Geometry check sheet. Reference: the model listing, model coordinates, mm. A direction names the side the tool comes from. Round coordinates to 2 decimals unless told otherwise and drop trailing zeros. Write each loop counter-clockwise with the first axis right and the second up, starting at its lowest first coordinate (ties: lowest second). Pieces come first, ordered by that corner, then holes. Notation, with made-up numbers: (67.5, 45) - (88.5, 45) arc R12 cw to (88.5, 55) - close; hole circle Ø9 at (-7, 88.5). An arc over 180 degrees is marked (long way). Return JSON: item names as keys, results as strings.
```python
from build123d import *

# Parameters (mm, degrees)
SKETCH1_R           = 56
BOSS_EXTRUDE1_DEPTH = 4
SKETCH2_R           = 4.5
CUT_EXTRUDE1_DEPTH  = 80.296910406
CUT_EXTRUDE2_DEPTH  = 80.296910406
SKETCH4_R           = 1
SKETCH4_R_2         = 1.5
CUT_EXTRUDE3_DEPTH  = 80.296910406


with BuildPart() as part:
    # Sketch1 → Boss-Extrude1 (new body)
    with BuildSketch(Plane(origin=(0, 0, 0), x_dir=(0, 0, -1), z_dir=(1, 0, 0))):
        Circle(SKETCH1_R)
    extrude(amount=BOSS_EXTRUDE1_DEPTH)

    # Sketch2 → Cut-Extrude1 (cut, through all)
    with BuildSketch(Plane.ZY):
        with Locations((0, 50)):
            Circle(SKETCH2_R)
        with Locations((43.301270189, -25)):
            Circle(SKETCH2_R)
        with Locations((-43.301270189, -25)):
            Circle(SKETCH2_R)
    extrude(amount=-CUT_EXTRUDE1_DEPTH, mode=Mode.SUBTRACT)

    # Sketch3 → Cut-Extrude2 (cut, through all)
    with BuildSketch(Plane.ZY):
        with BuildLine():
            Line((-30, -47.28636167), (-30, -37.28636167))
            Line((-30, -37.28636167), (30, -37.28636167))
            Line((30, -37.28636167), (30, -47.28636167))
            ThreePointArc((30, -47.28636167), (0, -56), (-30, -47.28636167))
        make_face()
    extrude(amount=-CUT_EXTRUDE2_DEPTH, mode=Mode.SUBTRACT)

    # Sketch4 → Cut-Extrude3 (cut, through all)
    with BuildSketch(Plane(origin=(4, 0, 0), x_dir=(0, 0, -1), z_dir=(1, 0, 0))):
        with Locations((-16.75, 39.058710316)):
            Circle(SKETCH4_R)
        with Locations((16.75, 39.058710316)):
            Circle(SKETCH4_R)
        with Locations((17.152725495, 21.063216097)):
            Circle(SKETCH4_R)
        with Locations((-16.347274505, 21.063216097)):
            Circle(SKETCH4_R)
        with Locations((-37, 15.884372564)):
            Circle(SKETCH4_R_2)
        with Locations((0, -16.070778671)):
            Circle(SKETCH4_R_2)
        with Locations((37, 15.884372564)):
            Circle(SKETCH4_R_2)
    extrude(amount=-CUT_EXTRUDE3_DEPTH, mode=Mode.SUBTRACT)


solid = part.part
```
(1) Release check for a two-part mould opening along Z. For faces 1 (the face through (1.972, 55.964, -2.019)), 2 (the face through (2, -42, 30)), 3 (the face through (0, 5, 1)) record: pulls with the +Z half, pulls with the -Z half, needs draft (parallel to the pull), parting line crosses it, or undercut.
Response values:
{"face 1": "parting line crosses it", "face 2": "undercut", "face 3": "needs draft"}
(2) Section check A-A, the plane z = 0. Enter the section's corners in (x, y).
Response values:
{"outline": "(0, -37.29) - (4, -37.29) - (4, -17.57) - (0, -17.57) - close; (0, -14.57) - (4, -14.57) - (4, 45.5) - (0, 45.5) - close; (0, 54.5) - (4, 54.5) - (4, 56) - (0, 56) - close"}
(3) Section check C-C, the plane x = 2.5. Give the number of separate pieces and of enclosed holes in the cut face, plus the area to 3 significant figures.
Response values:
{"separate pieces": "1", "enclosed holes": "10", "area": "8,670 mm^2"}
(4) Access from +Z, -Z, +X, -X, +Y, -Y to the whole of each face (thin tool, end or side, straight path). Record for faces 4 (the face through (1.97, 45.61, -0.98)), 5 (the face through (2, -42, -30)).
Response values:
{"face 4": "+X, -X", "face 5": "+X, -X, -Y"}
(5) Gauge pin test, flat ends, axial feed: pin 1 (5 mm diameter, centred on y = 8, z = -11, fed in from -X); pin 2 (2 mm diameter, centred on x = 2.5, y = -44, fed in from -Z); pin 3 (2 mm diameter, centred on x = 1.5, z = 32, fed in from +Y); pin 4 (2 mm diameter, centred on x = 1.5, y = 39, fed in from +Z). Record the tip position at first contact, or that the pin passes through.
Response values:
{"pin 1": "stops at x = 0", "pin 2": "stops at z = -35.87", "pin 3": "stops at y = 46.64", "pin 4": "stops at z = 41.13"}
(6) Material ranges on line 1 along Y through (x, z) = (3.7, -17); line 2 along Z through (x, y) = (2.85, -26); line 3 along Y through (x, z) = (1.75, -16.5), recorded low to high. Write a range as [from, to].
Response values:
{"line 1": "y = [-37.29, 20.07], [22.05, 38.09], [40.03, 53.36]", "line 2": "z = [-49.6, -47.69], [-38.91, 38.91], [47.69, 49.6]", "line 3": "y = [-37.29, 20.31], [21.82, 38.09], [40.03, 53.51]"}
(7) Section check D-D, the plane y = -25. Enter the section's corners in (x, z).
Response values:
{"outline": "(0, -50.11) - (4, -50.11) - (4, -47.8) - (0, -47.8) - close; (0, -38.8) - (4, -38.8) - (4, 38.8) - (0, 38.8) - close; (0, 47.8) - (4, 47.8) - (4, 50.11) - (0, 50.11) - close"}
(8) Section check B-B, the plane y = 50. Enter the section's corners in (x, z), plus the area to 3 significant figures.
Response values:
{"outline": "(0, -25.22) - (4, -25.22) - (4, -4.5) - (0, -4.5) - close; (0, 4.5) - (4, 4.5) - (4, 25.22) - (0, 25.22) - close", "area": "166 mm^2"}
